Input: part model. Units: mm. Frame: model coordinates. Face numbers are marked on the shaded views. A direction names the side the tool comes from. Coordinates: 2 decimals unless noted, no trailing zeros. Write each loop counter-clockwise with the first axis right and the second up, starting at its lowest first coordinate (ties: lowest second). Pieces come first, ordered by that corner, then holes.
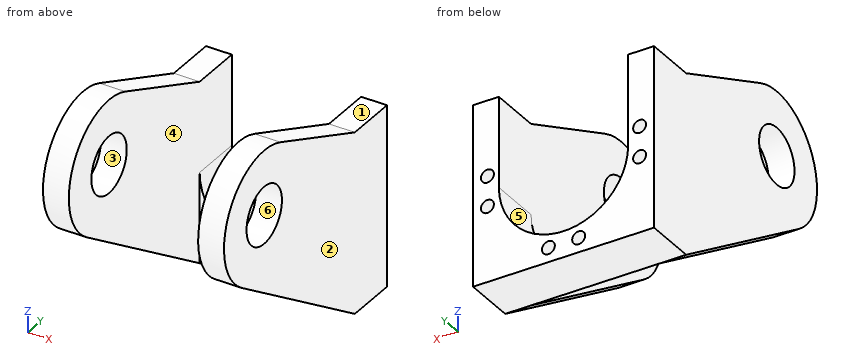
from build123d import *

# Parameters (mm, degrees)
SKETCH1_R               = 2.5
BOSS_EXTRUDE1_DEPTH     = 20
SKETCH7_R               = 25
SKETCH7_R_2             = 11
BOSS_EXTRUDE3_DEPTH     = 70
CUT_EXTRUDE8_DEPTH      = 102
CUT_EXTRUDE8_DEPTH_BACK = 102
SKETCH9_W               = 50
SKETCH9_H               = 83.625795222


with BuildPart() as part:
    # Sketch1 → Boss-Extrude1 (new body)
    with BuildSketch(Plane(origin=(0, 0, 0), x_dir=(1, 0, 0), z_dir=(0, 1, 0))):
        with BuildLine():
            Line((-35, 35), (-35, -35))
            Line((-35, -35), (-25, -35))
            Line((-25, -35), (-25, 0))
            ThreePointArc((-25, 0), (0, 25), (25, 0))
            Line((25, 0), (25, -35))
            Line((25, -35), (35, -35))
            Line((35, -35), (35, 35))
            Line((35, 35), (-35, 35))
        make_face()
        with Locations(Location((-29.423558412, -5.85270966, 0), (0, 0, 270))):
            Circle(SKETCH1_R, mode=Mode.SUBTRACT)
        with Locations(Location((29.423558412, -5.85270966, 0), (0, 0, 270))):
            Circle(SKETCH1_R, mode=Mode.SUBTRACT)
        with Locations(Location((-29.423558412, 5.85270966, 0), (0, 0, 270))):
            Circle(SKETCH1_R, mode=Mode.SUBTRACT)
        with Locations(Location((-5.85270966, 29.423558412, 0), (0, 0, 270))):
            Circle(SKETCH1_R, mode=Mode.SUBTRACT)
        with Locations(Location((29.423558412, 5.85270966, 0), (0, 0, 270))):
            Circle(SKETCH1_R, mode=Mode.SUBTRACT)
        with Locations(Location((5.85270966, 29.423558412, 0), (0, 0, 270))):
            Circle(SKETCH1_R, mode=Mode.SUBTRACT)
    extrude(amount=BOSS_EXTRUDE1_DEPTH)

    # Sketch7 → Boss-Extrude3 (add)
    # profile 1 of 2: a face of its own
    with BuildSketch(Plane(origin=(35, 0, 0), x_dir=(0, 0, -1), z_dir=(1, 0, 0))):
        with BuildLine():
            Line((-35, 0), (-55.374716919, -46.204663298))
            ThreePointArc((-55.374716919, -46.204663298), (-27.345774694, -31.828741331), (-7.5, -56.291651246))
            ThreePointArc((-7.5, -56.291651246), (-8.570053321, -63.527510003), (-11.688612156, -70.143948384))
            Line((-11.688612156, -70.143948384), (35, 0))
            Line((35, 0), (-35, 0))
        make_face()
    # profile 2 of 2: a face of its own
    with BuildSketch(Plane(origin=(35, 0, 0), x_dir=(0, 0, -1), z_dir=(1, 0, 0))):
        with Locations((-32.5, -56.291651246)):
            Circle(SKETCH7_R)
        with Locations((-32.5, -56.291651246)):
            Circle(SKETCH7_R_2, mode=Mode.SUBTRACT)
    extrude(amount=-BOSS_EXTRUDE3_DEPTH)

    # Sketch9 → Cut-Extrude8 (cut, two sides: drawn at the far end of the back side and taken through both)
    with BuildSketch(Plane.XY.offset(-CUT_EXTRUDE8_DEPTH_BACK)):
        with Locations((0, -41.812897611)):
            Rectangle(SKETCH9_W, SKETCH9_H)
    extrude(amount=CUT_EXTRUDE8_DEPTH + CUT_EXTRUDE8_DEPTH_BACK, mode=Mode.SUBTRACT)


solid = part.part
Item 1: Access query for the marked faces 1 and 2. Directions: +Z, -Z, +X, -X, +Y, -Y. A direction counts if a zero-diameter tool reaches every point of the face in a straight line with its end or side. Return the directions, or none.
Item 2: Section query A-A, the plane z = 32.5. Return loops of the section in (x, y), then the cut area to 3 significant figures.
Item 3: Section query B-B, the plane y = -59.5. Return loops of the section in (x, z).
Item 4: Pull-direction query (Z, two-part tool) for the marked faces 3, 4, 5 and 6; classes: released by +Z, released by -Z, zero draft, split by the parting line, or undercut.
Item 5: Section query C-C, the plane y = -73. Return loops of the section in (x, z), then the cut area to 3 significant figures.
Item 6: Material intervals for line 1 (Y direction, x = 33, z = 32.5); line 2 (X direction, y = -27, z = 37); line 3 (Y direction, x = 30, z = 27.5), sorted ascending.
Item 7: Pin query (flat end, axial travel): pin 1 Ø4 at (x, z) = (28.5, -5.5) entering from +Y; pin 2 Ø5 at (x, y) = (-23, 3) entering from +Z; pin 3 Ø2.5 at (x, z) = (29.5, 7) entering from +Y; pin 4 Ø8 at (x, z) = (29.42, 5.85) entering from -Y. Return the tip coordinate at first contact, or that it passes through.
Item 8: Section query D-D, the plane z = 5.5. Return loops of the section in (x, y).
The answers:
1. face 1: +Z, +X, -X, +Y
1. face 2: +Z, -Z, +X, +Y, -Y
2. outline: (-35, -81.29) - (-25, -81.29) - (-25, -67.29) - (-35, -67.29) - close; (-35, -45.29) - (-25, -45.29) - (-25, 20) - (-35, 20) - close; (25, -81.29) - (35, -81.29) - (35, -67.29) - (25, -67.29) - close; (25, -45.29) - (35, -45.29) - (35, 20) - (25, 20) - close
2. area: 1,590 mm2
3. outline: (-35, 4.6) - (-25, 4.6) - (-25, 21.98) - (-35, 21.98) - close; (-35, 43.02) - (-25, 43.02) - (-25, 57.29) - (-35, 57.29) - close; (25, 4.6) - (35, 4.6) - (35, 21.98) - (25, 21.98) - close; (25, 43.02) - (35, 43.02) - (35, 57.29) - (25, 57.29) - close
4. face 3: undercut
4. face 4: zero draft
4. face 5: released by +Z
4. face 6: undercut
5. outline: (-35, 13.9) - (-25, 13.9) - (-25, 51.1) - (-35, 51.1) - close; (25, 13.9) - (35, 13.9) - (35, 51.1) - (25, 51.1) - close
5. area: 744 mm2
6. line 1: y = -81.29 to -67.29, -45.29 to 20
6. line 2: x = -35 to -25, 25 to 35
6. line 3: y = -80.79 to -66.09, -46.49 to 20
7. pin 1: stops at y = 20
7. pin 2: stops at z = 35
7. pin 3: stops at y = 0
7. pin 4: stops at y = -67.38
8. outline: (-35, -60.85) - (-25, -60.85) - (-25, 20) - (-26.95, 20) - (-26.95, 0) - (-31.9, 0) - (-31.9, 20) - (-35, 20) - close; (25, -60.85) - (35, -60.85) - (35, 20) - (31.9, 20) - (31.9, 0) - (26.95, 0) - (26.95, 20) - (25, 20) - close
